```python
from build123d import *

# Parameters (mm, degrees)
F0_W     = 44.45
F0_H     = 1092.2
F1_DEPTH = 88.9
F2_W     = 38.1
F2_H     = 12.7
F3_DEPTH = 44.451
F4_R     = 5.08


with BuildPart() as f1:
    # F0 (on Front) → F1 (new body)
    with BuildSketch(Plane.XZ):
        with Locations((-22.225, 216.568415)):
            Rectangle(F0_W, F0_H)
    extrude(amount=F1_DEPTH)

    # F2 (on face) → F3 (cut, through all)
    with BuildSketch(Plane(origin=(-44.45, 0, 0), x_dir=(0, -1, 0), z_dir=(-1, 0, 0))):
        with Locations((44.45, 667.418415)):
            Rectangle(F2_W, F2_H)
        with Locations((44.45, -43.781585)):
            Rectangle(F2_W, F2_H)
        with Locations((44.45, 134.018415)):
            Rectangle(F2_W, F2_H)
        with Locations((44.45, 311.818415)):
            Rectangle(F2_W, F2_H)
        with Locations((44.45, -221.581585)):
            Rectangle(F2_W, F2_H)
        with Locations((44.45, 489.618415)):
            Rectangle(F2_W, F2_H)
    extrude(amount=-F3_DEPTH, mode=Mode.SUBTRACT)

    # F4
    f4_edges = [f1.edges().sort_by_distance(p)[0] for p in [
        (-44.45, -88.9, 216.568415),
        (0, -88.9, 216.568415),
        (-22.225, -88.9, 762.668415),
        (0, -44.45, 762.668415),
        (-44.45, -44.45, 762.668415),
        (-22.225, -88.9, -329.531585),
        (0, -44.45, -329.531585),
        (-44.45, -44.45, -329.531585),
    ]]
    fillet(f4_edges, radius=F4_R)


solid = f1.part
```
Verification items for the finished model (mm, model axes). A direction names the side the tool comes from. Coordinates: 2 decimals unless noted, no trailing zeros. Answer in a Markdown table with one row per item. Add a question column.
1. Access from +Z, -Z, +X, -X, +Y, -Y to the whole of each face (thin tool, end or side, straight path). Record for faces 4 (the face through (-23, -44, 305.468)), 5 (the face through (-44.45, -41, 209)).
2. Section check A-A, the plane y = -45.5. Give the number of separate pieces and of enclosed holes in the cut face, then the cut area to 3 significant figures.
3. Draft check along Y on faces 1 (the face through (-23, -44, 495.968)), 2 (the face through (-23, 0, 224)), 3 (the face through (-22, -41, 762.668)). Enter one of: +Y half, -Y half, draft (parallel to the pull), parting line (faces both ways), or undercut.
4. Material ranges on probe 1 along Z at (x, y) = (-5, -22.5); probe 2 along Y at (x, z) = (-17, 139); probe 3 along Z at (x, y) = (-43, -14), recorded low to high. Write a range as [from, to].
Derived:
| question | item | result |
|---|---|---|
| 1 | face 4 | +X, -X |
| 1 | face 5 | +Z, -Z, -X, +Y, -Y |
| 2 | separate pieces | 7 |
| 2 | enclosed holes | 0 |
| 2 | area | 45,100 mm² |
| 3 | face 1 | undercut |
| 3 | face 2 | +Y half |
| 3 | face 3 | draft |
| 4 | probe 1 | z = [-329.53, 762.67] |
| 4 | probe 2 | y = [-88.9, -63.5], [-25.4, 0] |
| 4 | probe 3 | z = [-328.01, 761.14] |
